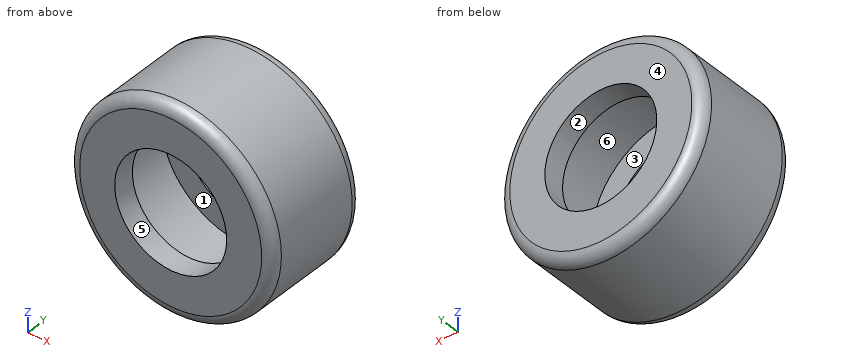
```python
from build123d import *

# Parameters (mm, degrees)
F0_R     = 47.741436
F0_R_2   = 26.252537
F1_DEPTH = 25.4
F2_R     = 5.08
F3_R     = 5.08
F4_T     = -10.16


with BuildPart() as f1:
    # F0 (on Front) → F1 (new body, symmetric)
    with BuildSketch(Plane.XZ):
        Circle(F0_R)
        Circle(F0_R_2, mode=Mode.SUBTRACT)
    extrude(amount=F1_DEPTH, both=True)

    # F2
    f2_edges = [f1.edges().sort_by_distance(p)[0] for p in [
        (-47.741436, -25.4, 0),
    ]]
    fillet(f2_edges, radius=F2_R)

    # F3
    f3_edges = [f1.edges().sort_by_distance(p)[0] for p in [
        (-47.741436, 25.4, 0),
    ]]
    fillet(f3_edges, radius=F3_R)

    # F4
    f4_openings = [f1.faces().sort_by_distance(p)[0] for p in [
        (-26.252537, 0, 0),
    ]]
    offset(amount=F4_T, openings=f4_openings)


solid = f1.part
```
CAD build for the part. Positions are in the model's coordinates, mm. Face numbers are marked on the shaded views. A direction names the side the tool comes from. Coordinates: 2 decimals unless noted, no trailing zeros. Order: outer loops, then holes, each group sorted by start corner. A loop starts at its lowest first (then second) coordinate and runs counter-clockwise, first axis right, second up. Notation, with made-up numbers: (45.5, -10) -> (69.5, -10) arc R5 ccw to (69.5, -1) -> close; hole circle Ø11 at (4, 1.25). An arc over 180 degrees is marked (long way). Use one line per item in the form item = value. Start each with the question number.
1) Band-saw the part on A-A on x = 0. Give the cut face in (y, z).
2) Band-saw the part on B-B on z = 0. Give the cut face in (x, y).
3) Band-saw the part on C-C on y = 10. Give the cut face in (x, z), then the cut area to 3 significant figures.
4) Drop flat-ended pins along their axis: pin 1 (5 mm diameter, centred on x = -26.5, z = -37, fed in from -Y); pin 2 (6 mm diameter, centred on x = 29, y = -11, fed in from +Z); pin 3 (1.5 mm diameter, centred on x = 13.5, y = -15, fed in from +Z). Give the stop position or say it passes through.
5) Pull direction Y, two halves, no side cores. Call the marked faces 1, 2, 3 and 4: +Y half, -Y half, draft (parallel to the pull), parting line (faces both ways), or undercut.
6) Drill centre lines: L1, parallel to Z at x = 0, y = -7; L2, parallel to Z at x = 0, y = -20; L3, parallel to Y at x = 20.5, z = 31. Where is each one in solid material? Low to high. Write a range as [from, to].
7) Tool access for the marked faces 5 and 6: list every direction of +Z, -Z, +X, -X, +Y, -Y with a clear straight run to the whole face (end or side of a thin tool).
8) Band-saw the part on D-D on y = 22.5. Give the cut face in (x, z), then the cut area to 3 significant figures.
Entries:
q1.outline = (-25.4, -42.66) arc R5.08 ccw to (-20.32, -47.74) -> (20.32, -47.74) arc R5.08 ccw to (25.4, -42.66) -> (25.4, -26.25) -> (15.24, -26.25) -> (15.24, -37.58) -> (-15.24, -37.58) -> (-15.24, -26.25) -> (-25.4, -26.25) -> close; (-25.4, 26.25) -> (-15.24, 26.25) -> (-15.24, 37.58) -> (15.24, 37.58) -> (15.24, 26.25) -> (25.4, 26.25) -> (25.4, 42.66) arc R5.08 ccw to (20.32, 47.74) -> (-20.32, 47.74) arc R5.08 ccw to (-25.4, 42.66) -> close
q2.outline = (-47.74, -20.32) arc R5.08 ccw to (-42.66, -25.4) -> (-26.25, -25.4) -> (-26.25, -15.24) -> (-37.58, -15.24) -> (-37.58, 15.24) -> (-26.25, 15.24) -> (-26.25, 25.4) -> (-42.66, 25.4) arc R5.08 ccw to (-47.74, 20.32) -> close; (26.25, -25.4) -> (42.66, -25.4) arc R5.08 ccw to (47.74, -20.32) -> (47.74, 20.32) arc R5.08 ccw to (42.66, 25.4) -> (26.25, 25.4) -> (26.25, 15.24) -> (37.58, 15.24) -> (37.58, -15.24) -> (26.25, -15.24) -> close
q3.outline = circle Ø95.48 at (0, 0); hole circle Ø75.16 at (0, 0)
q3.area = 2,720 mm2
q4.pin_1 = -25.39
q4.pin_2 = 40.04
q4.pin_3 = 46.01
q5.face_1 = undercut
q5.face_2 = draft
q5.face_3 = undercut
q5.face_4 = +Y half
q6.L1 = [-47.74, -37.58], [37.58, 47.74]
q6.L2 = [-47.74, -26.25], [26.25, 47.74]
q6.L3 = [-25.4, -15.24], [15.24, 25.4]
q7.face_5 = +Y, -Y
q7.face_6 = none
q8.outline = circle Ø94.5 at (0, 0); hole circle Ø52.51 at (0, 0)
q8.area = 4,850 mm2
